Input: part model. Units: mm. Frame: model coordinates. Coordinates: 2 decimals unless noted, no trailing zeros. Loops run counter-clockwise (first coordinate to the right, second up) from the corner with the lowest first, then second, coordinate; pieces in that order, holes last. Notation, with made-up numbers: (77.5, -6) -> (98.5, -6) arc R8 ccw to (98.5, -2) -> close; hole circle Ø9 at (-20.75, -28.75). An arc over 180 degrees is marked (long way). Answer as a JSON object with one key per item and string values.
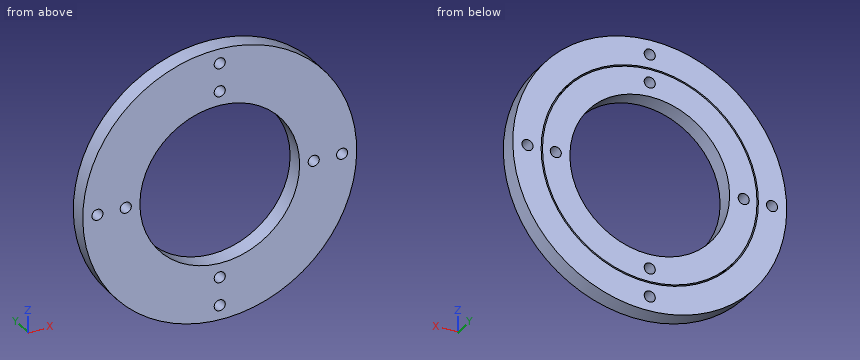
from build123d import *

# Parameters (mm, degrees)
SKETCH_1_R          = 60
SKETCH_1_R_2        = 35
EXTRUDE_1_DEPTH     = 8
SKETCH_2_R          = 47.6
SKETCH_2_R_2        = 47
CUT_EXTRUDE_1_DEPTH = 7.5
SKETCH_3_R          = 2.425
CUT_EXTRUDE_2_DEPTH = 86.229103011
SKETCH_4_R          = 2.425
CUT_EXTRUDE_3_DEPTH = 86.229103011


with BuildPart() as part:
    # 草图1 → 凸台-拉伸1 (new body)
    with BuildSketch(Plane(origin=(0, 0, 0), x_dir=(1, 0, 0), z_dir=(0, 1, 0))):
        with Locations(Location((0, 0, 0), (0, 0, 270))):
            Circle(SKETCH_1_R)
        with Locations(Location((0, 0, 0), (0, 0, 270))):
            Circle(SKETCH_1_R_2, mode=Mode.SUBTRACT)
    extrude(amount=EXTRUDE_1_DEPTH)

    # 草图2 → 切除-拉伸1 (cut)
    with BuildSketch(Plane(origin=(0, 8, 0), x_dir=(1, 0, 0), z_dir=(0, 1, 0))):
        with Locations(Location((0, 0, 0), (0, 0, 270))):
            Circle(SKETCH_2_R)
        with Locations(Location((0, 0, 0), (0, 0, 270))):
            Circle(SKETCH_2_R_2, mode=Mode.SUBTRACT)
    extrude(amount=-CUT_EXTRUDE_1_DEPTH, mode=Mode.SUBTRACT)

    # 草图3 → 切除-拉伸2 (cut, through all)
    with BuildSketch(Plane(origin=(0, 8, 0), x_dir=(1, 0, 0), z_dir=(0, 1, 0))):
        with BuildLine():
            ThreePointArc((-43.6, 0), (-41.175, -2.425), (-38.75, 0))
            Line((-38.75, 0), (-43.6, 0))
        make_face()
        with BuildLine():
            Line((-43.6, 0), (-38.75, 0))
            ThreePointArc((-38.75, 0), (-41.175, 2.425), (-43.6, 0))
        make_face()
        with Locations(Location((0, 41.175, 0), (0, 0, 270))):
            Circle(SKETCH_3_R)
        with BuildLine():
            ThreePointArc((43.6, 0), (41.175, 2.425), (38.75, 0))
            Line((38.75, 0), (43.6, 0))
        make_face()
        with BuildLine():
            Line((43.6, 0), (38.75, 0))
            ThreePointArc((38.75, 0), (41.175, -2.425), (43.6, 0))
        make_face()
        with Locations(Location((0, -41.175, 0), (0, 0, 270))):
            Circle(SKETCH_3_R)
    extrude(amount=-CUT_EXTRUDE_2_DEPTH, mode=Mode.SUBTRACT)

    # 草图4 → 切除-拉伸3 (cut, through all)
    with BuildSketch(Plane(origin=(0, 8, 0), x_dir=(1, 0, 0), z_dir=(0, 1, 0))):
        with Locations(Location((0, 53.575, 0), (0, 0, 270))):
            Circle(SKETCH_4_R)
        with Locations(Location((53.575, 0, 0), (0, 0, 270))):
            Circle(SKETCH_4_R)
        with Locations(Location((0, -53.575, 0), (0, 0, 270))):
            Circle(SKETCH_4_R)
        with BuildLine():
            ThreePointArc((-56, 0), (-53.575, -2.425), (-51.15, 0))
            Line((-51.15, 0), (-56, 0))
        make_face()
        with BuildLine():
            Line((-56, 0), (-51.15, 0))
            ThreePointArc((-51.15, 0), (-53.575, 2.425), (-56, 0))
        make_face()
    extrude(amount=-CUT_EXTRUDE_3_DEPTH, mode=Mode.SUBTRACT)


solid = part.part
1. Pin query (flat end, axial travel): P1, Ø1.5, axis at y = 1, z = 1, coming from the -X side; P2, Ø3, axis at y = 6, z = -26.5, coming from the +X side. Return the tip coordinate at first contact, or that it passes through.
Reply:
{"P1": "stops at x = -60", "P2": "stops at x = 54.54"}
2. Section query D-D (z = 19.5). Return loops of the section in (x, y).
Reply:
{"outline": "(-56.74, 0) -> (-29.06, 0) -> (-29.06, 8) -> (-42.76, 8) -> (-42.76, 0.5) -> (-43.42, 0.5) -> (-43.42, 8) -> (-56.74, 8) -> close; (29.06, 0) -> (56.74, 0) -> (56.74, 8) -> (43.42, 8) -> (43.42, 0.5) -> (42.76, 0.5) -> (42.76, 8) -> (29.06, 8) -> close"}
3. Section query A-A (x = 0). Count the separate pieces of the cut face and the enclosed holes in it, plus the area to 3 significant figures.
Reply:
{"separate pieces": "6", "enclosed holes": "0", "area": "236 mm2"}
4. Line query: line 1 along Z through (x, y) = (-4.5, 6.5); line 2 along Z through (x, y) = (29, 4.75); line 3 along X through (y, z) = (2, 32). Output: solid intervals per line, ascending.
Reply:
{"line 1": "z = -59.83 to -47.39, -46.78 to -34.71, 34.71 to 46.78, 47.39 to 59.83", "line 2": "z = -52.53 to -37.75, -36.99 to -19.6, 19.6 to 36.99, 37.75 to 52.53", "line 3": "x = -50.75 to -35.24, -34.42 to -14.18, 14.18 to 34.42, 35.24 to 50.75"}
